Verification items for the finished model (mm, model axes). Give positions to 0.01 mm unless a question says otherwise; leave off trailing zeros. Loops run counter-clockwise (first coordinate to the right, second up) from the corner with the lowest first, then second, coordinate; pieces in that order, holes last. Notation, with made-up numbers: (78.25, 18.25) - (137.25, 18.25) arc R31 cw to (137.25, 49.25) - close; hole circle Ø11 at (-16, -34.75). An arc over 180 degrees is marked (long way). Answer in a Markdown table with one row per item.
```python
from build123d import *

# Parameters (mm, degrees)
SKETCH1_R                                       = 15.875
BOSS_EXTRUDE1_DEPTH                             = 1
CUT_EXTRUDE1_DEPTH                              = 23.472900347
CUT_EXTRUDE1_DEPTH_BACK                         = 23.472900347
SKETCH2_R                                       = 7.5
CUT_EXTRUDE2_DEPTH                              = 23.472900347
CUT_EXTRUDE2_DEPTH_BACK                         = 23.472900347
SKETCH4_R                                       = 0.25
CSK_FOR_M2_FLAT_HEAD_MACHINE_SCREW1_D           = 1
CSK_FOR_M2_FLAT_HEAD_MACHINE_SCREW1_CSINK_D     = 1.6
CSK_FOR_M2_FLAT_HEAD_MACHINE_SCREW1_CSINK_ANGLE = 100


with BuildPart() as part:
    # Sketch1 → Boss-Extrude1 (new body)
    with BuildSketch(Plane(origin=(0, 0, 0), x_dir=(1, 0, 0), z_dir=(0, 1, 0))):
        with Locations(Location((0, 0, 0), (0, 0, 270))):
            Circle(SKETCH1_R)
    extrude(amount=BOSS_EXTRUDE1_DEPTH)

    # Sketch2 → Cut-Extrude1 (cut, two sides: drawn at the far end of the back side and taken through both)
    with BuildSketch(Plane(origin=(0, 1, 0), x_dir=(1, 0, 0), z_dir=(0, 1, 0)).offset(-CUT_EXTRUDE1_DEPTH_BACK)):
        with Locations(Location((0, 0, 0), (0, 0, 270))):
            Circle(SKETCH2_R)
    extrude(amount=CUT_EXTRUDE1_DEPTH + CUT_EXTRUDE1_DEPTH_BACK, mode=Mode.SUBTRACT)

    # Sketch4 → Cut-Extrude2 (cut, two sides: drawn at the far end of the back side and taken through both)
    with BuildSketch(Plane(origin=(0, 1, 0), x_dir=(1, 0, 0), z_dir=(0, 1, 0)).offset(-CUT_EXTRUDE2_DEPTH_BACK)):
        with Locations(Location((0, 10.25, 0), (0, 0, 270))):
            Circle(SKETCH4_R)
    extrude(amount=CUT_EXTRUDE2_DEPTH + CUT_EXTRUDE2_DEPTH_BACK, mode=Mode.SUBTRACT)

    # CSK for M2 Flat Head Machine Screw1 (through all)
    with Locations(Plane(origin=(0, 1, 0), x_dir=(1, 0, 0), z_dir=(0, 1, 0))):
        with Locations((0, 14.29), (14.29, 0), (0, -14.29), (-14.29, 0)):
            CounterSinkHole(CSK_FOR_M2_FLAT_HEAD_MACHINE_SCREW1_D / 2, CSK_FOR_M2_FLAT_HEAD_MACHINE_SCREW1_CSINK_D / 2, counter_sink_angle=CSK_FOR_M2_FLAT_HEAD_MACHINE_SCREW1_CSINK_ANGLE)


solid = part.part
```
Q1. Sectioned sample at B-B (y = 0.25). Record the cut outline in (x, z) (3 decimals), and give its area (3 significant figures).
Completed:
| item | result |
|---|---|
| outline | circle Ø31.75 at (0, 0); hole circle Ø1 at (-14.29, 0); hole circle Ø15 at (0, 0); hole circle Ø1 at (0, -14.29); hole circle Ø1 at (0, 14.29); hole circle Ø0.5 at (0, -10.25); hole circle Ø1 at (14.29, 0) |
| area | 612 mm^2 |
Q2. Thickness scan on line 1 (Z direction, x = 5, y = 0.7); line 2 (X direction, y = 0.4, z = 14.29); line 3 (X direction, y = 0.2, z = 5.5). Record the ranges inside material, lowest first.
Completed:
| item | result |
|---|---|
| line 1 | -15.07 to -5.59, 5.59 to 15.07 |
| line 2 | -6.91 to -0.5, 0.5 to 6.91 |
| line 3 | -14.89 to -5.1, 5.1 to 14.89 |
Q3. Sectioned sample at D-D (z = -7). Record the cut outline in (x, y).
Completed:
| item | result |
|---|---|
| outline | (-14.25, 0) - (-2.69, 0) - (-2.69, 1) - (-14.25, 1) - close; (2.69, 0) - (14.25, 0) - (14.25, 1) - (2.69, 1) - close |
Q4. Sectioned sample at A-A (z = 0). Record the cut outline in (x, y) (3 decimals), and give its area (3 significant figures).
Completed:
| item | result |
|---|---|
| outline | (-15.875, 0) - (-14.79, 0) - (-14.79, 0.748) - (-15.09, 1) - (-15.875, 1) - close; (-13.79, 0) - (-7.5, 0) - (-7.5, 1) - (-13.49, 1) - (-13.79, 0.748) - close; (7.5, 0) - (13.79, 0) - (13.79, 0.748) - (13.49, 1) - (7.5, 1) - close; (14.79, 0) - (15.875, 0) - (15.875, 1) - (15.09, 1) - (14.79, 0.748) - close |
| area | 14.6 mm^2 |
Q5. Draft check along Z on faces 1 (the face through (0.1, 0.4, 13.8)), 2 (the face through (-7, 1, -4)), 3 (the face through (-15.497, 0.493, -3.441)). Enter one of: +Z half, -Z half, draft (parallel to the pull), parting line (faces both ways), or undercut.
Completed:
| item | result |
|---|---|
| face 1 | undercut |
| face 2 | draft |
| face 3 | parting line |
Q6. Sectioned sample at C-C (x = 14.29). Record the cut outline in (y, z).
Completed:
| item | result |
|---|---|
| outline | (0, -6.91) - (1, -6.91) - (1, -0.8) - (0.75, -0.5) - (0, -0.5) - close; (0, 0.5) - (0.75, 0.5) - (1, 0.8) - (1, 6.91) - (0, 6.91) - close |
